Geometry: final body of the model. Coordinates: model frame, mm. A direction names the side the tool comes from. Give positions to 0.01 mm unless a question says otherwise; leave off trailing zeros. Write each loop counter-clockwise with the first axis right and the second up, starting at its lowest first coordinate (ties: lowest second). Pieces come first, ordered by that corner, then holes. Notation, with made-up numbers: (88.25, 4) - (133.25, 4) arc R20 ccw to (133.25, 23) - close; hole circle Ø1 at (30, -24.5). An arc over 180 degrees is marked (long way). Use CSV: the item, a comma, the result in double quotes. Start each with the question number.
(1) Reachability of faces 1 (the flat face through (10.671, 13.147, -0.07)), 2 (the flat face through (-9.88, 14.11, -0.07)), 3 (the cylindrical face through (-2.88, 0.05, -0.64)) from +Z, -Z, +X, -X, +Y, -Y: full face, straight path, thin tool, end or side. Return the list, or none.
(2) Section A-A on y = 0. Output: boundary loops of the cut face in (x, z), and give its area (3 significant figures).
(3) Line query: probe 1 along X at (y, z) = (0, 0); probe 2 along X at (y, z) = (-12.5, 1); probe 3 along Y at (x, z) = (-11, 0.25). Output: solid intervals per line, ascending. Write a range as [from, to].
(4) First-contact query: pin 1 Ø0.8 at (x, z) = (-4.5, 1) entering from +Y; pin 2 Ø1.5 at (x, z) = (-6, -0.5) entering from -Y; pin 3 Ø0.6 at (x, z) = (4, -1) entering from +Y; pin 4 Ø12 at (x, y) = (5.5, 8.5) entering from -Z. Flat tips, straight axial feed; report the tip coordinate or a pass-through.
(5) Draft query along Y for faces 4 (the flat face through (-5, -14, -5)), 5 (the cylindrical face through (-0.48, -14.29, 3.26)), 6 (the flat face through (-10.648, 13.114, -0.07)), 7 (the flat face through (0, 16, 0)). Return one class per face: released by +Y, released by -Y, zero draft, split by the parting line, or undercut.
(6) Section B-B on y = 11.5. Output: boundary loops of the cut face in (x, z).
from build123d import *

# Parameters (mm, degrees)
BOSS_EXTRUDE1_DEPTH             = 5
BOSS_EXTRUDE1_DEPTH_BACK        = 5
SKETCH2_R                       = 2.95
BOSS_EXTRUDE2_DEPTH             = 16
BOSS_EXTRUDE2_DIRECTION_2_REACH = 24.483
FILLET2_R                       = 2
FILLET3_R                       = 2


with BuildPart() as part:
    # Sketch1 → Boss-Extrude1 (new, two sides: drawn at the far end of the back side and taken through both)
    with BuildSketch(Plane.XY.offset(-BOSS_EXTRUDE1_DEPTH_BACK)):
        with BuildLine():
            Line((8.20214304, 11.713874233), (10.467878905, 14.949680393))
            ThreePointArc((10.467878905, 14.949680393), (10.974647974, 14.627825025), (11.471528727, 14.290904731))
            Line((11.471528727, 14.290904731), (9.846733622, 11.970456841))
            ThreePointArc((9.846733622, 11.970456841), (0, -15.5), (-9.846733622, 11.970456841))
            Line((-9.846733622, 11.970456841), (-11.471528727, 14.290904731))
            ThreePointArc((-11.471528727, 14.290904731), (-10.974647974, 14.627825025), (-10.467878905, 14.949680393))
            Line((-10.467878905, 14.949680393), (-8.20214304, 11.713874233))
            ThreePointArc((-8.20214304, 11.713874233), (0, -14.3), (8.20214304, 11.713874233))
        make_face()
    extrude(amount=BOSS_EXTRUDE1_DEPTH + BOSS_EXTRUDE1_DEPTH_BACK)

    # Sketch2 → Boss-Extrude2 (add)
    with BuildSketch(Plane(origin=(0, 0, 0), x_dir=(1, 0, 0), z_dir=(0, 1, 0))):
        with Locations(Location((0, 0, 0), (0, 0, 270))):
            Circle(SKETCH2_R)
    extrude(amount=BOSS_EXTRUDE2_DEPTH)

    # Sketch2 → Boss-Extrude2 direction 2 (add, up to next)
    with BuildSketch(Plane(origin=(0, 0, 0), x_dir=(1, 0, 0), z_dir=(0, 1, 0)), mode=Mode.PRIVATE) as boss_extrude2_direction_2_sk1:
        with Locations(Location((0, 0, 0), (0, 0, 270))):
            Circle(SKETCH2_R)
    boss_extrude2_direction_2_tool1 = extrude(boss_extrude2_direction_2_sk1.sketch, amount=-BOSS_EXTRUDE2_DIRECTION_2_REACH, mode=Mode.PRIVATE) - part.part
    add(boss_extrude2_direction_2_tool1.solids().sort_by_distance((0, 0, 0))[0])

    # Fillet2
    fillet2_edges = [part.edges().sort_by_distance(p)[0] for p in [
        (0, 16, -2.95),
    ]]
    fillet(fillet2_edges, radius=FILLET2_R)

    # Fillet3
    fillet3_edges = [part.edges().sort_by_distance(p)[0] for p in [
        (-8.20214304, 11.713874233, 0),
        (8.20214304, 11.713874233, 0),
    ]]
    fillet(fillet3_edges, radius=FILLET3_R)

    # Sketch4 → Revolve1 (revolve)
    with BuildSketch(Plane(origin=(0, 0, 0), x_dir=(0, 0, -1), z_dir=(1, 0, 0))):
        with BuildLine():
            Line((0, -14.986224552), (-4.696335741, -14.986224552))
            ThreePointArc((-4.696335741, -14.986224552), (-2.444681768, -15.973915756), (0, -16.236614408))
            Line((0, -16.236614408), (0, -14.986224552))
        make_face()
    revolve(axis=Axis((0, -14.986224552, 0), (0, 1, 0)))


solid = part.part
Check values:
1,face 1,"+Z, -Z, +X"
1,face 2,"+Z, -Z, +Y"
1,face 3,"+Y"
2,outline,"(-15.5, -5) - (-14.3, -5) - (-14.3, 5) - (-15.5, 5) - close; circle Ø5.9 at (0, 0); (14.3, -5) - (15.5, -5) - (15.5, 5) - (14.3, 5) - close"
2,area,"51.3 mm²"
3,probe 1,"x = [-15.5, -14.3], [-2.95, 2.95], [14.3, 15.5]"
3,probe 2,"x = [-9.17, -6.95], [-2.78, 2.78], [6.95, 9.17]"
3,probe 3,"y = [-10.92, -9.14], [9.14, 10.92], [13.62, 14.61]"
4,pin 1,"stops at y = -13.43"
4,pin 2,"stops at y = -14.58"
4,pin 3,"stops at y = -13.64"
4,pin 4,"stops at z = -5"
5,face 4,"zero draft"
5,face 5,"undercut"
5,face 6,"undercut"
5,face 7,"released by +Y"
6,outline,"(-10.39, -5) - (-9.01, -5) - (-9.01, 5) - (-10.39, 5) - close; circle Ø5.9 at (0, 0); (9.01, -5) - (10.39, -5) - (10.39, 5) - (9.01, 5) - close"
